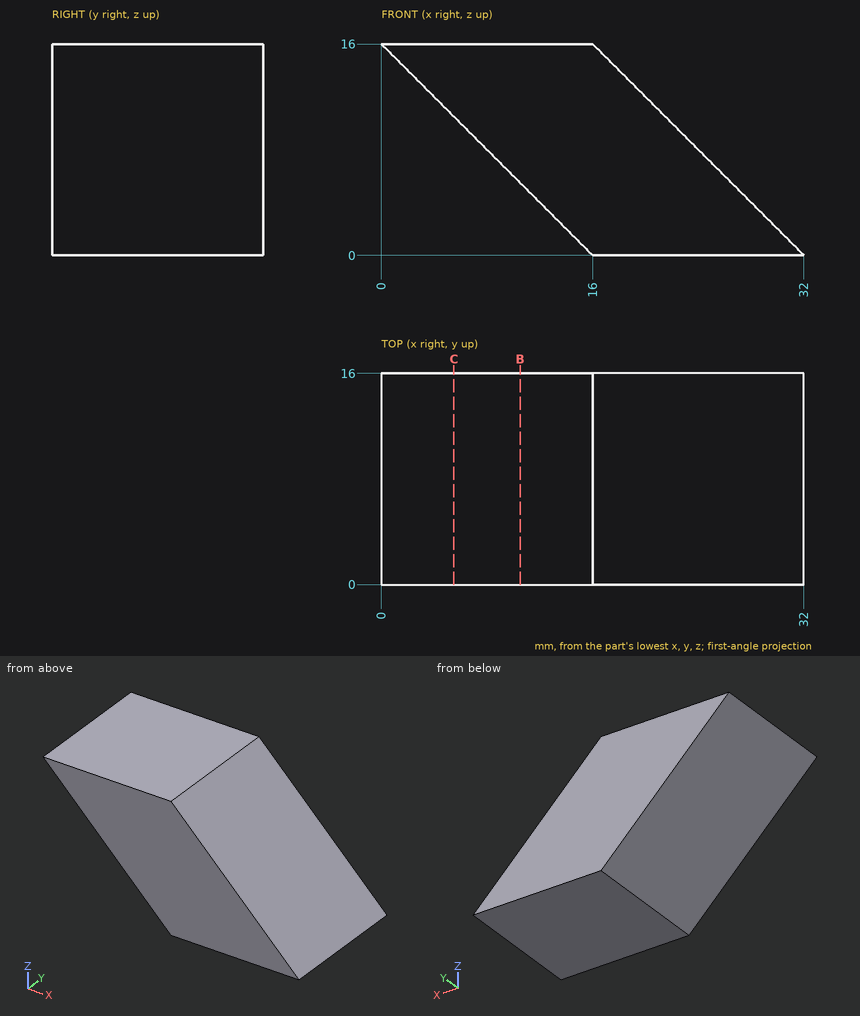
Verification items for this drawing (mm, ordinates from the low corner). Coordinates: 2 decimals unless noted, no trailing zeros. Write each loop counter-clockwise with the first axis right and the second up, starting at its lowest first coordinate (ties: lowest second). Pieces come first, ordered by that corner, then holes. Notation, with made-up numbers: M -29,6.5 L -12,6.5 A17 ccw -12,33.5 Z; hole C 10,77 d2. An arc over 180 degrees is marked long. Answer as a JSON object with one key per item and string values. Group by question number.
(1) Cross-section at C-C, the plane x = 5.5. Record the cut outline in (y, z).
(2) Gauge pin test, flat ends, axial feed: pin 1 (1.5 mm diameter, centred on y = 11.5, z = 7, fed in from -X); pin 2 (3 mm diameter, centred on x = 24, y = 3, fed in from +Z); pin 3 (4 mm diameter, centred on y = 10.5, z = 5, fed in from -X). Record the tip position at first contact, or that the pin passes through.
(3) Material ranges on line 1 (X direction, y = 3.75, z = 3); line 2 (X direction, y = 14.75, z = 7.75); line 3 (Z direction, x = 19, y = 4), recorded low to high.
(4) Cross-section at B-B, the plane x = 10.5. Record the cut outline in (y, z), and give its area (3 significant figures).
Reply:
{
 "1": {"outline": "M 0,10.5 L 16,10.5 L 16,16 L 0,16 Z"},
 "2": {"pin 1": "x = 8.25", "pin 2": "z = 9.5", "pin 3": "x = 9"},
 "3": {"line 1": "13 to 29", "line 2": "8.25 to 24.25", "line 3": "0 to 13"},
 "4": {"outline": "M 0,5.5 L 16,5.5 L 16,16 L 0,16 Z", "area": "168 mm²"}
}
